from build123d import *

# Parameters (mm, degrees)
BOSS_EXTRUDE1_DEPTH = 19.5
SKETCH2_R           = 24.75
BOSS_EXTRUDE2_DEPTH = 17.5
SKETCH3_R           = 22.25
BOSS_EXTRUDE3_DEPTH = 14
FILLET1_SIZE        = 2.5
SKETCH4_R           = 1.25
SKETCH4_R_2         = 1.025
CUT_EXTRUDE1_DEPTH  = 6


with BuildPart() as part:
    # Sketch1 → Boss-Extrude1 (new body)
    with BuildSketch(Plane(origin=(0, 0, 0), x_dir=(1, 0, 0), z_dir=(0, 1, 0))):
        with BuildLine():
            Line((-16.75, -27.75), (16.75, -27.75))
            ThreePointArc((16.75, -27.75), (24.528174593, -24.528174593), (27.75, -16.75))
            Line((27.75, -16.75), (27.75, 16.75))
            ThreePointArc((27.75, 16.75), (24.528174593, 24.528174593), (16.75, 27.75))
            Line((16.75, 27.75), (-16.75, 27.75))
            ThreePointArc((-16.75, 27.75), (-24.528174593, 24.528174593), (-27.75, 16.75))
            Line((-27.75, 16.75), (-27.75, -16.75))
            ThreePointArc((-27.75, -16.75), (-24.528174593, -24.528174593), (-16.75, -27.75))
        make_face()
    extrude(amount=BOSS_EXTRUDE1_DEPTH)

    # Sketch2 → Boss-Extrude2 (add)
    with BuildSketch(Plane(origin=(0, 19.5, 0), x_dir=(1, 0, 0), z_dir=(0, 1, 0))):
        with Locations(Location((0, 0, 0), (0, 0, 270))):
            Circle(SKETCH2_R)
    extrude(amount=BOSS_EXTRUDE2_DEPTH)

    # Sketch3 → Boss-Extrude3 (add)
    with BuildSketch(Plane(origin=(0, 37, 0), x_dir=(1, 0, 0), z_dir=(0, 1, 0))):
        with Locations(Location((0, 0, 0), (0, 0, 270))):
            Circle(SKETCH3_R)
    extrude(amount=BOSS_EXTRUDE3_DEPTH)

    # Fillet1
    fillet1_edges = [part.edges().sort_by_distance(p)[0] for p in [
        (0, 37, -22.25),
        (0, 51, -22.25),
    ]]
    chamfer(fillet1_edges, length=FILLET1_SIZE - 0.0001)  # a hair under: the kernel refuses the full size

    # Sketch4 → Cut-Extrude1 (cut)
    with BuildSketch(Plane.XZ):
        with Locations(Location((21.5, 21.5, 0), (0, 0, 270))):
            Circle(SKETCH4_R)
        with Locations(Location((25, 0, 0), (0, 0, 270))):
            Circle(SKETCH4_R_2)
        with Locations(Location((21.5, -21.5, 0), (0, 0, 90))):
            Circle(SKETCH4_R)
        with Locations(Location((-21.5, -21.5, 0), (0, 0, 270))):
            Circle(SKETCH4_R)
        with Locations(Location((-25, 0, 0), (0, 0, 90))):
            Circle(SKETCH4_R_2)
        with Locations(Location((-21.5, 21.5, 0), (0, 0, 90))):
            Circle(SKETCH4_R)
    extrude(amount=-CUT_EXTRUDE1_DEPTH, mode=Mode.SUBTRACT)


solid = part.part
Work out the finished part from the listing and answer in its coordinate system (mm). A direction names the side the tool comes from. Give positions to 0.01 mm unless a question says otherwise; leave off trailing zeros. Order: outer loops, then holes, each group sorted by start corner. A loop starts at its lowest first (then second) coordinate and runs counter-clockwise, first axis right, second up. Notation, with made-up numbers: (60, -23.75) -> (84, -23.75) arc R28 ccw to (84, -2.75) -> close; hole circle Ø6 at (83, 52.5). An arc over 180 degrees is marked (long way). Answer as a JSON object with one key per item and string values. Group by question number.
1. Consider line 1 along X through (y, z) = (4, -21.5); line 2 along Z through (x, y) = (21, 1); line 3 along Z through (x, y) = (-25, 1.2) (3 decimals). Determine where each line is inside the solid, lowest interval first. Write a range as [from, to].
2. Section B-B on y = 47 is taken. Determine the outline of the cut face in (x, z).
3. Section C-C on y = 32 is taken. Determine the outline of the cut face in (x, z).
4. A tool of negligible diameter and unlimited length cuts with its end or side. For faces 1 (the flat face through (-25, 19.5, 0)), 2 (the cylindrical face through (24.613, 9.614, -24.442)), 3 (the flat face through (-25, 6, 0)), from which of +Z, -Z, +X, -X, +Y, -Y can it reach the whole face along a straight path? Write none if from no direction.
5. The mould has two halves that part along X. Classify faces 4 (the cylindrical face through (24.442, 9.614, 24.613)), 5 (the conical face through (5.97, 50.88, 18.95)), 6 (the cylindrical face through (21.979, 2.958, -20.345)): released by +X, released by -X, zero draft, split by the parting line, or undercut.
6. Flat-ended cylindrical pins translate along their axes: pin 1 Ø1.5 at (x, z) = (-21.5, -21.5) entering from +Y; pin 2 Ø3 at (y, z) = (25.5, 17) entering from +X; pin 3 Ø3.5 at (x, z) = (-25, 0) entering from +Y; pin 4 Ø2 at (x, z) = (22, 21.5) entering from -Y. Find the tip coordinate at first contact, or state that the pin passes through.
Result sheet:
{
 "1": {"line 1": "x = [-26.67, -22.75], [-20.25, 20.25], [22.75, 26.67]", "line 2": "z = [-26.9, -22.65], [-20.35, 20.35], [22.65, 26.9]", "line 3": "z = [-24.026, -1.025], [1.025, 24.026]"},
 "2": {"outline": "circle Ø44.5 at (0, 0)"},
 "3": {"outline": "circle Ø49.5 at (0, 0)"},
 "4": {"face 1": "+Y", "face 2": "-Z, +X, +Y, -Y", "face 3": "-Y"},
 "5": {"face 4": "released by +X", "face 5": "split by the parting line", "face 6": "undercut"},
 "6": {"pin 1": "stops at y = 19.5", "pin 2": "stops at x = 19.3", "pin 3": "stops at y = 38.5", "pin 4": "stops at y = 0"}
}
